The model under review builds one solid part; all positions refer to its coordinate system, in mm. A direction names the side the tool comes from. Round coordinates to 2 decimals unless told otherwise and drop trailing zeros. Order: outer loops, then holes, each group sorted by start corner. A loop starts at its lowest first (then second) coordinate and runs counter-clockwise, first axis right, second up. Notation, with made-up numbers: M 34.5,79.5 L 83.5,79.5 A8 ccw 83.5,93.5 Z; hole C 33.25,47 d6. An arc over 180 degrees is marked long. Answer as a JSON object with one key per item and string values. Group by question number.
1) Consider section D-D, the plane y = -31. Write out the cut boundary in (x, z).
2) To check wall thickness, follow line 1 (Y direction, x = 0, z = 4); line 2 (Y direction, x = 0, z = 1.5); line 3 (Y direction, x = 0, z = 6.75). State the ranges of each line that lie inside material, in increasing order.
3) Consider section B-B, the plane y = -10. Write out the cut boundary in (x, z).
4) For faces 1 (the flat face through (1, -21, 4)), 2 (the flat face through (-2, -24, 8)), 3 (the cylindrical face through (-3.86, -5.9, 0.79)), list the 3-axis set-ups (+Z, -Z, +X, -X, +Y, -Y) from which the entire face can be reached by the end or side of a thin tool; tool diameter is ignored.
5) Consider section A-A, the plane x = 0. Write out the cut boundary in (y, z).
6) Consider section C-C, the plane x = 3.75. Write out the cut boundary in (y, z).
7) The part is to be moulded in two halves that separate along X. For faces 4 (the flat face through (1, -13.5, 5)), 5 (the cylindrical face through (0.215, -29.364, 3.178)), 6 (the flat face through (5, -33, 4)), say which applies: +X half, -X half, draft (parallel to the pull), parting line (faces both ways), or undercut.
8) Insertion check: pin 1 Ø4 at (x, y) = (1, -17) entering from +Z; pin 2 Ø2.5 at (y, z) = (-17.5, 2.5) entering from +X. Each pin has a flat end and moves straight along its axis. Give the tip position at first contact, or say it passes through.
```python
from build123d import *

# Parameters (mm, degrees)
SKETCH099_R         = 1.32
PAD061_DEPTH        = 8
POCKET030_DEPTH     = 1.6
HOLE006_D           = 3.3
HOLE006_CSINK_D     = 6
HOLE006_CSINK_ANGLE = 82


with BuildPart() as part:
    # Sketch099 → Pad061 (new body)
    with BuildSketch(Plane.XY):
        Polygon((-7, -44), (5, -44), (5, -21), (-3, -21), (-3, -13.5), (5, -13.5), (5, -5), (-7, -5), align=None)
        with Locations((0, -10)):
            Circle(SKETCH099_R, mode=Mode.SUBTRACT)
    extrude(amount=PAD061_DEPTH)

    # Sketch100 → Pocket030 (cut)
    with BuildSketch(Plane.XY):
        with BuildLine():
            Line((6, -21), (-3, -21))
            Line((-3, -21), (-3, -8))
            ThreePointArc((-3, -8), (-3.87868, -5.87868), (-6, -5))
            Line((-6, -5), (-6, 4))
            Line((-6, 4), (6, 4))
            Line((6, 4), (6, -21))
        make_face()
    extrude(amount=POCKET030_DEPTH, mode=Mode.SUBTRACT)

    # Hole006 (through all)
    with Locations(Plane.XY.offset(8)):
        with Locations((0, -31), (0, -39)):
            CounterSinkHole(HOLE006_D / 2, HOLE006_CSINK_D / 2, counter_sink_angle=HOLE006_CSINK_ANGLE)


solid = part.part
```
Results list:
{
 "1": {"outline": "M -7,0 L -1.65,0 L -1.65,6.45 L -3,8 L -7,8 Z; M 1.65,0 L 5,0 L 5,8 L 3,8 L 1.65,6.45 Z"},
 "2": {"line 1": "-44 to -40.65, -37.35 to -32.65, -29.35 to -21, -13.5 to -11.32, -8.68 to -5", "line 2": "-44 to -40.65, -37.35 to -32.65, -29.35 to -21", "line 3": "-44 to -40.91, -37.09 to -32.91, -29.09 to -21, -13.5 to -11.32, -8.68 to -5"},
 "3": {"outline": "M -7,0 L -3,0 L -3,1.6 L -1.32,1.6 L -1.32,8 L -7,8 Z; M 1.32,1.6 L 5,1.6 L 5,8 L 1.32,8 Z"},
 "4": {"face 1": "+Z, -Z, +X", "face 2": "+Z, +X, -X, +Y, -Y", "face 3": "-Z, +X, +Y"},
 "5": {"outline": "M -44,0 L -40.65,0 L -40.65,6.45 L -42,8 L -44,8 Z; M -37.35,0 L -32.65,0 L -32.65,6.45 L -34,8 L -36,8 L -37.35,6.45 Z; M -29.35,0 L -21,0 L -21,8 L -28,8 L -29.35,6.45 Z; M -13.5,1.6 L -11.32,1.6 L -11.32,8 L -13.5,8 Z; M -8.68,1.6 L -5,1.6 L -5,8 L -8.68,8 Z"},
 "6": {"outline": "M -44,0 L -21,0 L -21,8 L -44,8 Z; M -13.5,1.6 L -5,1.6 L -5,8 L -13.5,8 Z"},
 "7": {"face 4": "draft", "face 5": "undercut", "face 6": "+X half"},
 "8": {"pin 1": "through", "pin 2": "x = -3"}
}
